The drawing under review shows one solid part. Ordinate dimensions are in mm from its lowest x, y, z. A direction names the side the tool comes from. Give positions to 0.01 mm unless a question says otherwise; leave off trailing zeros. Loops run counter-clockwise (first coordinate to the right, second up) from the corner with the lowest first, then second, coordinate; pieces in that order, holes last. Notation, with made-up numbers: (26.5, -14.5) - (85.5, -14.5) arc R26 ccw to (85.5, 17.5) - close; hole circle Ø4 at (15.25, 77). An arc over 180 degrees is marked (long way). Write each question's results on one line, items separated by ' | '.
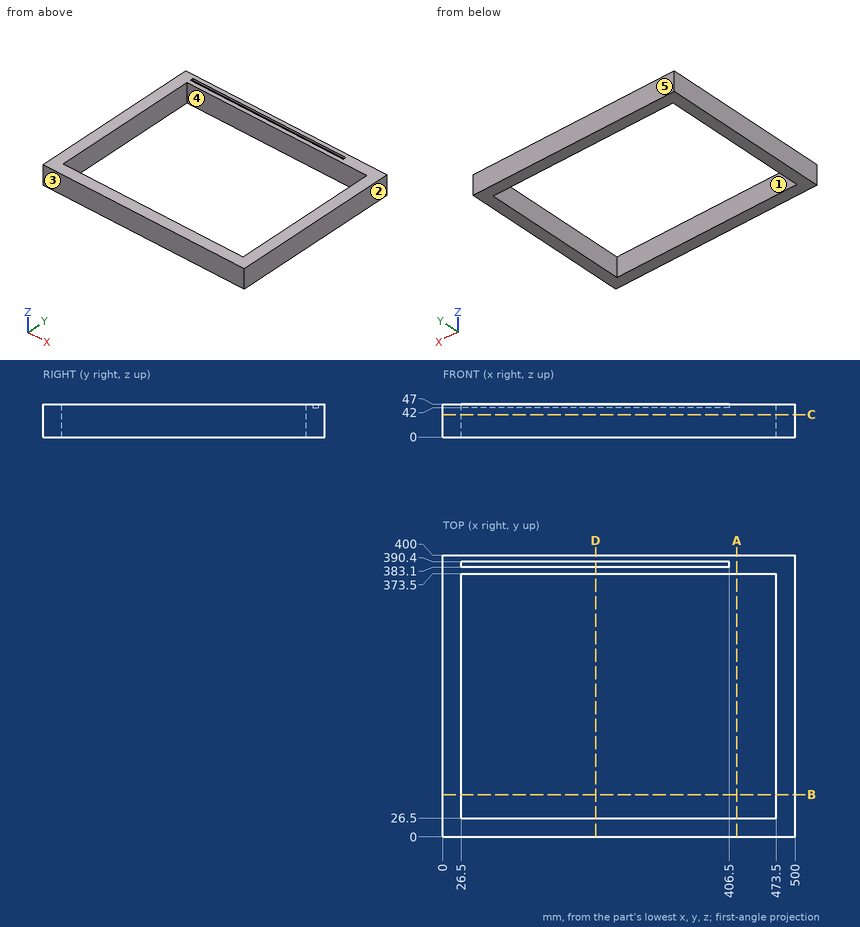
(1) Take a section at C-C on z = 32. Give the boundary of the cut face in (x, y).
Answers below:
outline: (0, 0) - (500, 0) - (500, 400) - (0, 400) - close; hole (26.5, 26.5) - (473.5, 26.5) - (473.5, 373.5) - (26.5, 373.5) - close
(2) Take a section at A-A on x = 417.5. Give the boundary of the cut face in (y, z), plus the area to 3 significant figures.
Answers below:
outline: (0, 0) - (26.5, 0) - (26.5, 47) - (0, 47) - close; (373.5, 0) - (400, 0) - (400, 47) - (373.5, 47) - close | area: 2,490 mm2
(3) Draft analysis for pull direction Y (two halves, no side actions). For the marked faces 3, 4 and 5, state which applies: pulls with the +Y half, pulls with the -Y half, needs draft (parallel to the pull), parting line crosses it, or undercut.
Answers below:
face 3: pulls with the -Y half | face 4: undercut | face 5: pulls with the +Y half
(4) Tool access review of the marked faces 1 and 2: name each direction out of +Z, -Z, +X, -X, +Y, -Y from which nothing blocks a thin tool from reaching the whole face with its end or side.
Answers below:
face 1: +Z, -Z | face 2: +Z, -Z, +X, +Y, -Y
(5) Take a section at B-B on y = 60. Give the boundary of the cut face in (x, z), plus the area to 3 significant figures.
Answers below:
outline: (0, 0) - (26.5, 0) - (26.5, 47) - (0, 47) - close; (473.5, 0) - (500, 0) - (500, 47) - (473.5, 47) - close | area: 2,490 mm2
(6) Wall thickness on line 1 along Y through (x, z) = (384, 42.5); line 2 along Y through (x, z) = (303.5, 29); line 3 along X through (y, z) = (45, 3): over which ranges is each line inside the solid? List them lowest first. Write a range as from..to.
Answers below:
line 1: 0..26.5, 373.5..383.1, 390.4..400 | line 2: 0..26.5, 373.5..400 | line 3: 0..26.5, 473.5..500
(7) Insertion check: P1, Ø2, axis at x = 271.5, y = 387, coming from the +Z side. The pin has a flat end and moves straight along its axis. Give the tip position at first contact, or say it passes through.
Answers below:
P1: z = 42
(8) Take a section at D-D on x = 217. Give the boundary of the cut face in (y, z).
Answers below:
outline: (0, 0) - (26.5, 0) - (26.5, 47) - (0, 47) - close; (373.5, 0) - (400, 0) - (400, 47) - (390.4, 47) - (390.4, 42) - (383.1, 42) - (383.1, 47) - (373.5, 47) - close
